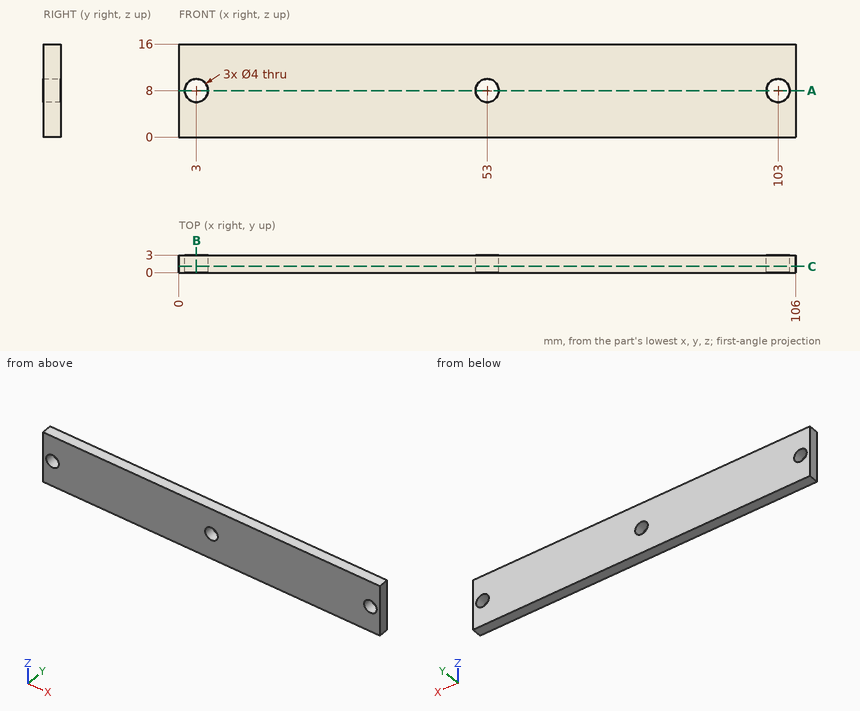
Here's the drawing with two shaded views (mm, measured from the low corner). I have some questions. Round coordinates to 2 decimals unless told otherwise and drop trailing zeros. Loops run counter-clockwise (first coordinate to the right, second up) from the corner with the lowest first, then second, coordinate; pieces in that order, holes last.
1. Suppose I cut it at B-B, the plane x = 3. Please give me the cut outline in (y, z).
Answers:
outline: (0, 0) - (3, 0) - (3, 6) - (0, 6) - close; (0, 10) - (3, 10) - (3, 16) - (0, 16) - close
2. If I drill on probe 1 along X at (y, z) = (1.7, 8); probe 2 along Z at (x, y) = (3, 2.45); probe 3 along Z at (x, y) = (53.5, 1.8), over which ranges is the centre line in solid material (lowest first)?
Answers:
probe 1: x = 0 to 1, 5 to 51, 55 to 101, 105 to 106
probe 2: z = 0 to 6, 10 to 16
probe 3: z = 0 to 6.06, 9.94 to 16
3. Suppose I cut it at A-A, the plane z = 8. Please give me the cut outline in (x, y), and give its area (3 significant figures).
Answers:
outline: (0, 0) - (1, 0) - (1, 3) - (0, 3) - close; (5, 0) - (51, 0) - (51, 3) - (5, 3) - close; (55, 0) - (101, 0) - (101, 3) - (55, 3) - close; (105, 0) - (106, 0) - (106, 3) - (105, 3) - close
area: 282 mm2
4. Suppose I cut it at C-C, the plane y = 1.05. Please give me the cut outline in (x, z).
Answers:
outline: (0, 0) - (106, 0) - (106, 16) - (0, 16) - close; hole circle Ø4 at (3, 8); hole circle Ø4 at (53, 8); hole circle Ø4 at (103, 8)
5. Will this pin go through, and if not, where does the flat tip stop? pin 1 (1.5 mm diameter, centred on y = 1.5, z = 5, fed in from -X).
Answers:
pin 1: stops at x = 0
